from build123d import *

# Parameters (mm, degrees)
SKETCH1_R           = 9.525
BOSS_EXTRUDE1_DEPTH = 14.06
SKETCH2_R           = 6.35
BOSS_EXTRUDE2_DEPTH = 16.94
SKETCH3_W           = 1.59
SKETCH3_H           = 5.56
CUT_EXTRUDE1_DEPTH  = 8.47
SKETCH5_R           = 1.19
CUT_EXTRUDE3_DEPTH  = 14.06
SKETCH4_R           = 5.555
CUT_EXTRUDE4_DEPTH  = 14.06


with BuildPart() as part:
    # Sketch1 → Boss-Extrude1 (new body)
    with BuildSketch(Plane(origin=(0, 0, 0), x_dir=(1, 0, 0), z_dir=(0, 1, 0))):
        with Locations(Location((0, 0, 0), (0, 0, 270))):
            Circle(SKETCH1_R)
    extrude(amount=BOSS_EXTRUDE1_DEPTH)



with BuildPart() as body_2:
    # Sketch2 → Boss-Extrude2 (new body)
    with BuildSketch(Plane(origin=(0, 38.1, 0), x_dir=(1, 0, 0), z_dir=(0, 1, 0))):
        with Locations(Location((0, 0, 0), (0, 0, 270))):
            Circle(SKETCH2_R)
    extrude(amount=-BOSS_EXTRUDE2_DEPTH)


with BuildPart() as part_1:
    add(part.part)

    add(body_2.part)  # loft1 joins it to this body
    # loft up to a face of the part (loft1)
    loft([Face(Wire([part_1.edges().sort_by_distance((6.943426176, 14.06, -6.520311184))[0]])), Face(Wire([part_1.edges().sort_by_distance((-4.628950784, 21.16, -4.346874123))[0]]))])

    # Sketch3 → Cut-Extrude1 (cut, symmetric)
    with BuildSketch(Plane.XY):
        with Locations((5.555, 35.32)):
            Rectangle(SKETCH3_W, SKETCH3_H)
    extrude(amount=CUT_EXTRUDE1_DEPTH, both=True, mode=Mode.SUBTRACT)

    # Sketch5 → Cut-Extrude3 (cut)
    with BuildSketch(Plane(origin=(0, 0, 0), x_dir=(0, 0, -1), z_dir=(1, 0, 0))):
        with Locations(Location((0, 6.35, 0), (0, 0, 180))):
            Circle(SKETCH5_R)
    extrude(amount=CUT_EXTRUDE3_DEPTH, mode=Mode.SUBTRACT)

    # Sketch4 → Cut-Extrude4 (cut)
    with BuildSketch(Plane.XZ):
        with Locations(Location((-0.795, -0.79, 0), (0, 0, 270))):
            Circle(SKETCH4_R)
    extrude(amount=-CUT_EXTRUDE4_DEPTH, mode=Mode.SUBTRACT)


solid = part_1.part
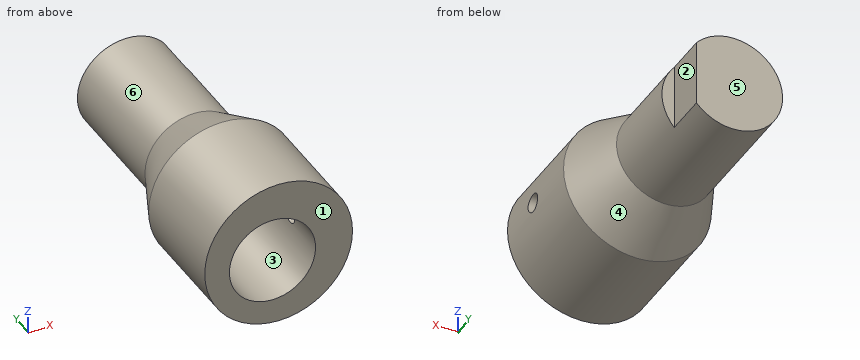
Could you check a few things on this model? Use its own coordinates, in mm. Face numbers are marked on the shaded views. A direction names the side the tool comes from. Give positions to 0.01 mm unless a question says otherwise; leave off trailing zeros. Loops run counter-clockwise (first coordinate to the right, second up) from the corner with the lowest first, then second, coordinate; pieces in that order, holes last. Notation, with made-up numbers: (73, 14) -> (87, 14) arc R9 ccw to (87, 18) -> close; hole circle Ø6 at (-5, 24.5). An arc over 180 degrees is marked (long way). Return JSON: item names as keys, results as strings.
Item 1: Which directions (+Z, -Z, +X, -X, +Y, -Y) give clear straight access to the entire face, cutting with the end or side of a thin tool? Please do the marked faces 5 and 6.
Geometry results:
{"face 5": "+Z, -Z, +X, -X, +Y", "face 6": "+Y"}
Item 2: If we section it at D-D on y = 35: List the corners of the cut face in (x, z) for me, plus the area to 3 significant figures.
Geometry results:
{"outline": "(4.76, -4.2) -> (4.76, 4.2) arc R6.35 ccw (long way) to start", "area": "118 mm²"}
Item 3: I'm going to push flat-ended pins straight in: pin 1 (1 mm diameter, centred on x = 5, y = 4, fed in from -Z) (3 decimals); pin 2 (6 mm diameter, centred on y = 20.5, z = 5, fed in from -X); pin 3 (1.7 mm diameter, centred on y = 36, z = -2, fed in from +X). Where does each tip first touch, or does it pass through?
Geometry results:
{"pin 1": "stops at z = -8.395", "pin 2": "stops at x = -7.03", "pin 3": "stops at x = 4.76"}
Item 4: We'd pull the mould along X, two halves only. Please class the marked faces 1, 2, 3 and 4: +X half, -X half, draft (parallel to the pull), parting line (faces both ways), or undercut.
Geometry results:
{"face 1": "draft", "face 2": "+X half", "face 3": "undercut", "face 4": "parting line"}
Item 5: If we section it at C-C on y = 13: List the corners of the cut face in (x, z) for me (3 decimals), plus the area to 3 significant figures.
Geometry results:
{"outline": "circle Ø19.05 at (0, 0); hole circle Ø11.11 at (-0.795, -0.79)", "area": "188 mm²"}
Item 6: If we section it at B-B on y = 30: List the corners of the cut face in (x, z) for me.
Geometry results:
{"outline": "circle Ø12.7 at (0, 0)"}
Item 7: I need wall thicknesses on L1, parallel to X at y = 9, z = -0.79; L2, parallel to Y at x = -2, z = 0; L3, parallel to Z at x = 5.75, y = 6.35. Which ranges of each line are inside material? Lowest first, please. Write a range as from..to.
Geometry results:
{"L1": "x = -9.49..-6.35, 4.76..9.49", "L2": "y = 14.06..38.1", "L3": "z = -7.59..-1.19, 1.19..7.59"}
Item 8: If we section it at A-A on z = 0: List the corners of the cut face in (x, y) for me (3 decimals), plus the area to 3 significant figures.
Geometry results:
{"outline": "(-9.525, 0) -> (-6.294, 0) -> (-6.294, 14.06) -> (4.704, 14.06) -> (4.704, 7.54) -> (9.525, 7.54) -> (9.525, 14.06) -> (6.35, 21.16) -> (6.35, 32.54) -> (4.76, 32.54) -> (4.76, 38.1) -> (-6.35, 38.1) -> (-6.35, 21.16) -> (-9.525, 14.06) -> close; (4.704, 0) -> (9.525, 0) -> (9.525, 5.16) -> (4.704, 5.16) -> close", "area": "421 mm²"}
